from build123d import *

# Parameters (mm, degrees)
SKETCH1_R                    = 17.8
BOSS_EXTRUDE1_DEPTH          = 57.5
SKETCH2_R                    = 5.65
BOSS_EXTRUDE2_DEPTH          = 4.5
SKETCH3_R                    = 1.585
BOSS_EXTRUDE3_DEPTH          = 16.5
F_3_0_3_DIAMETER_HOLE1_D     = 3
F_3_0_3_DIAMETER_HOLE1_DEPTH = 6.35
F_3_0_3_DIAMETER_HOLE1_TIP   = 0.901290929


with BuildPart() as part:
    # Sketch1 → Boss-Extrude1 (new body)
    with BuildSketch(Plane.XY):
        Circle(SKETCH1_R)
    extrude(amount=BOSS_EXTRUDE1_DEPTH)

    # Sketch2 → Boss-Extrude2 (add)
    with BuildSketch(Plane.XY.offset(57.5)):
        Circle(SKETCH2_R)
    extrude(amount=BOSS_EXTRUDE2_DEPTH)

    # Sketch3 → Boss-Extrude3 (add)
    with BuildSketch(Plane.XY.offset(62)):
        Circle(SKETCH3_R)
    extrude(amount=BOSS_EXTRUDE3_DEPTH)

    # Ø3.0 (3) Diameter Hole1
    with Locations(Plane.XY.offset(57.5)):
        with Locations((0, 12.446), (0, -12.5)):
            Hole(F_3_0_3_DIAMETER_HOLE1_D / 2, depth=F_3_0_3_DIAMETER_HOLE1_DEPTH)
            with Locations((0, 0, -(F_3_0_3_DIAMETER_HOLE1_DEPTH + F_3_0_3_DIAMETER_HOLE1_TIP / 2))):  # 118° drill point
                Cone(0, F_3_0_3_DIAMETER_HOLE1_D / 2, F_3_0_3_DIAMETER_HOLE1_TIP, mode=Mode.SUBTRACT)


solid = part.part
Source: CAD feature listing. Evaluate the final solid. Frame: model axes, mm. A direction names the side the tool comes from. Give positions to 0.01 mm unless a question says otherwise; leave off trailing zeros. Order: outer loops, then holes, each group sorted by start corner. A loop starts at its lowest first (then second) coordinate and runs counter-clockwise, first axis right, second up. Notation, with made-up numbers: (74.5, 28.25) -> (124.5, 28.25) arc R20 ccw to (124.5, 42.25) -> close; hole circle Ø11 at (7.5, 75). An arc over 180 degrees is marked (long way). Use a Markdown table: item, result.
1) Section query B-B, the plane x = 4. Return the cut outline in (y, z), then the cut area to 3 significant figures.
Answer list:
| item | result |
|---|---|
| outline | (-17.34, 0) -> (17.34, 0) -> (17.34, 57.5) -> (3.99, 57.5) -> (3.99, 62) -> (-3.99, 62) -> (-3.99, 57.5) -> (-17.34, 57.5) -> close |
| area | 2,030 mm² |
2) Section query A-A, the plane y = 0. Return the cut outline in (x, z) (3 decimals).
Answer list:
| item | result |
|---|---|
| outline | (-17.8, 0) -> (17.8, 0) -> (17.8, 57.5) -> (5.65, 57.5) -> (5.65, 62) -> (1.585, 62) -> (1.585, 78.5) -> (-1.585, 78.5) -> (-1.585, 62) -> (-5.65, 62) -> (-5.65, 57.5) -> (-17.8, 57.5) -> close |
3) Mould query, pull axis X, two halves, no side actions, for faces 3 (the conical face through (0.12, 12.21, 50.41)), 4 (the flat face through (-1.3, -1.2, 62)), 5 (the cylindrical face through (5.39, 1.7, 59.72)). Classes: +X half, -X half, draft (parallel to the pull), parting line (faces both ways), or undercut.
Answer list:
| item | result |
|---|---|
| face 3 | undercut |
| face 4 | draft |
| face 5 | parting line |
4) Section query D-D, the plane x = -3. Return the cut outline in (y, z).
Answer list:
| item | result |
|---|---|
| outline | (-17.55, 0) -> (17.55, 0) -> (17.55, 57.5) -> (4.79, 57.5) -> (4.79, 62) -> (-4.79, 62) -> (-4.79, 57.5) -> (-17.55, 57.5) -> close |
5) Contact query for flat-ended pins moving along their axis: P1, Ø10.5, axis at x = 5.5, y = 6, coming from the +Z side; P2, Ø6, axis at y = 12.5, z = 14, coming from the +X side; P3, Ø3, axis at y = -9, z = 48, coming from the -X side; P4, Ø6, axis at y = 7.5, z = 66, coming from the -X side. Output: stop coordinate, or through.
Answer list:
| item | result |
|---|---|
| P1 | z = 62 |
| P2 | x = 15.05 |
| P3 | x = -16.14 |
| P4 | through |
6) Ray query, line 1 along Y through (x, z) = (0, 54); line 2 along Z through (x, y) = (6.5, -12.5); line 3 along Y through (x, z) = (0.5, 66.5). Return the intervals inside material, ascending. Write a range as [from, to].
Answer list:
| item | result |
|---|---|
| line 1 | [-17.8, -14], [-11, 10.95], [13.95, 17.8] |
| line 2 | [0, 57.5] |
| line 3 | [-1.5, 1.5] |
7) Section query C-C, the plane z = 65. Return the cut outline in (x, y) (3 decimals), then the cut area to 3 significant figures.
Answer list:
| item | result |
|---|---|
| outline | circle Ø3.17 at (0, 0) |
| area | 7.89 mm² |
8) Reachability of faces 1 (the flat face through (0, 0, 78.5)), 2 (the cylindrical face through (0, -14, 54)) from +Z, -Z, +X, -X, +Y, -Y: full face, straight path, thin tool, end or side. Return the list, or none.
Answer list:
| item | result |
|---|---|
| face 1 | +Z, +X, -X, +Y, -Y |
| face 2 | +Z |
